CAD build for the part. Positions are in the model's coordinates, mm. A direction names the side the tool comes from. Coordinates: 2 decimals unless noted, no trailing zeros. Order: outer loops, then holes, each group sorted by start corner. A loop starts at its lowest first (then second) coordinate and runs counter-clockwise, first axis right, second up. Notation, with made-up numbers: (24, -25.75) - (38, -25.75) arc R21 ccw to (38, 6.25) - close; hole circle Ø9 at (55, 49). An arc over 180 degrees is marked (long way). Return JSON: item names as keys, results as strings.
from build123d import *

# Parameters (mm, degrees)
F0_W      = 93
F0_H      = 70
F0_R      = 1.5
F0_H_2    = 17
F0_R_2    = 3.25
F0_W_2    = 6
F0_H_3    = 6
F0_R_3    = 6
F0_W_3    = 14
F0_H_4    = 12
F0_R_4    = 3.5
F0_R_5    = 1.75
F1_DEPTH  = 1.5
F2_W      = 20.3
F2_H      = 8.7
F2_W_2    = 18.3
F2_H_2    = 6.7
F3_DEPTH  = 9
F2_W_3    = 26
F2_H_3    = 26.35
F4_DEPTH  = 3.5
F5_DEPTH  = 18.5
F6_DEPTH  = 6
F2_W_4    = 50
F2_H_4    = 1.5
F7_DEPTH  = 4
F8_DEPTH  = 10
F9_DEPTH  = 3.5
F10_DEPTH = 6.7
F11_DEPTH = 27
F12_DEPTH = 17
F13_DEPTH = 14
F14_DEPTH = 7
F15_DEPTH = 8
F16_W     = 6
F16_H     = 43
F17_DEPTH = 3.5
F18_DEPTH = 8
F19_R     = 1
F21_DEPTH = 1
F22_W     = 2.2
F22_H     = 24
F23_DEPTH = 10


with BuildPart() as f1:
    # F0 (on Front) → F1 (new body)
    with BuildSketch(Plane.XZ):
        with Locations((46.5, 52)):
            Rectangle(F0_W, F0_H)
        with Locations((2.5, 19.5)):
            Circle(F0_R, mode=Mode.SUBTRACT)
        with Locations((90.5, 19.5)):
            Circle(F0_R, mode=Mode.SUBTRACT)
        with Locations((2.5, 84.5)):
            Circle(F0_R, mode=Mode.SUBTRACT)
        with Locations((90.5, 84.5)):
            Circle(F0_R, mode=Mode.SUBTRACT)
        with Locations((46.5, 8.5)):
            Rectangle(F0_W, F0_H_2)
        with Locations((8.5, 11.5)):
            Circle(F0_R_2, mode=Mode.SUBTRACT)
        with Locations((50, 8)):
            Rectangle(F0_W_2, F0_H_3, mode=Mode.SUBTRACT)
        with Locations((65.5, 8)):
            Circle(F0_R_3, mode=Mode.SUBTRACT)
        with Locations((83, 8)):
            Rectangle(F0_W_3, F0_H_4, mode=Mode.SUBTRACT)
        with Locations((83, 8)):
            Rectangle(F0_W_3, F0_H_4)
        with Locations((83, 8)):
            Circle(F0_R_4, mode=Mode.SUBTRACT)
        with Locations((65.5, 8)):
            Circle(F0_R_3)
        with Locations((83, 8)):
            Circle(F0_R_4)
        with BuildLine():
            ThreePointArc((80.4019237886, 6.5), (82.2235428647, 10.8977774789), (86, 8))
            ThreePointArc((86, 8), (85.8977774789, 7.2235428647), (85.5980762114, 6.5))
            ThreePointArc((85.5980762114, 6.5), (83, 5), (80.4019237886, 6.5))
        make_face(mode=Mode.SUBTRACT)
        with Locations((50, 8)):
            Rectangle(F0_W_2, F0_H_3)
        with Locations((50, 8)):
            Circle(F0_R_5, mode=Mode.SUBTRACT)
        with Locations((8.5, 11.5)):
            Circle(F0_R_2)
        with BuildLine():
            ThreePointArc((85.5980762114, 6.5), (85.8977774789, 7.2235428647), (86, 8))
            ThreePointArc((86, 8), (82.2235428647, 10.8977774789), (80.4019237886, 6.5))
            Line((80.4019237886, 6.5), (85.5980762114, 6.5))
        make_face()
        with Locations((50, 8)):
            Circle(F0_R_5)
        with BuildLine():
            Line((85.5980762114, 6.5), (80.4019237886, 6.5))
            ThreePointArc((80.4019237886, 6.5), (83, 5), (85.5980762114, 6.5))
        make_face()
    extrude(amount=-F1_DEPTH)

    # F2 (on face) → F3 (join)
    with BuildSketch(Plane(origin=(0, 1.5, 0), x_dir=(-1, 0, 0), z_dir=(0, 1, 0))):
        with Locations((-61.75, 76.05)):
            Rectangle(F2_W, F2_H)
        with Locations((-61.75, 76.05)):
            Rectangle(F2_W_2, F2_H_2, mode=Mode.SUBTRACT)
        with Locations((-31.25, 76.05)):
            Rectangle(F2_W, F2_H)
        with Locations((-31.25, 76.05)):
            Rectangle(F2_W_2, F2_H_2, mode=Mode.SUBTRACT)
    extrude(amount=F3_DEPTH)

    # F2 (on face) → F4 (join)
    with BuildSketch(Plane(origin=(0, 1.5, 0), x_dir=(-1, 0, 0), z_dir=(0, 1, 0))):
        with Locations((-13, 51.525)):
            Rectangle(F2_W_3, F2_H_3)
    extrude(amount=F4_DEPTH)

    # F5 (add): faces of the model
    f5_faces = [f1.faces().sort_by_distance(p)[0] for p in [
        (61.75, 1.5, 76.05),
        (31.25, 1.5, 76.05),
    ]]
    extrude(f5_faces, amount=F5_DEPTH)

    # F0 (on Front) → F6 (join)
    with BuildSketch(Plane.XZ):
        with Locations((46.5, 52)):
            Rectangle(F0_W, F0_H)
        with Locations((2.5, 19.5)):
            Circle(F0_R, mode=Mode.SUBTRACT)
        with Locations((90.5, 19.5)):
            Circle(F0_R, mode=Mode.SUBTRACT)
        with Locations((2.5, 84.5)):
            Circle(F0_R, mode=Mode.SUBTRACT)
        with Locations((90.5, 84.5)):
            Circle(F0_R, mode=Mode.SUBTRACT)
    extrude(amount=F6_DEPTH)

    # F2 (on face) → F7 (join)
    with BuildSketch(Plane(origin=(0, 1.5, 0), x_dir=(-1, 0, 0), z_dir=(0, 1, 0))):
        with Locations((-38, 19.5)):
            Rectangle(F2_W_4, F2_H_4)
    extrude(amount=F7_DEPTH)

    # F0 (on Front) → F8 (join)
    with BuildSketch(Plane.XZ):
        with Locations((65.5, 8)):
            Circle(F0_R_3)
    extrude(amount=F8_DEPTH)

    # F0 (on Front) → F9 (join)
    with BuildSketch(Plane.XZ):
        with Locations((50, 8)):
            Rectangle(F0_W_2, F0_H_3)
        with Locations((50, 8)):
            Circle(F0_R_5, mode=Mode.SUBTRACT)
    extrude(amount=F9_DEPTH)

    # F0 (on Front) → F10 (join)
    with BuildSketch(Plane.XZ):
        with Locations((50, 8)):
            Circle(F0_R_5)
    extrude(amount=F10_DEPTH)

    # F0 (on Front) → F11 (join)
    with BuildSketch(Plane.XZ):
        with BuildLine():
            ThreePointArc((85.5980762114, 6.5), (85.8977774789, 7.2235428647), (86, 8))
            ThreePointArc((86, 8), (82.2235428647, 10.8977774789), (80.4019237886, 6.5))
            Line((80.4019237886, 6.5), (85.5980762114, 6.5))
        make_face()
    extrude(amount=F11_DEPTH)

    # F0 (on Front) → F12 (join)
    with BuildSketch(Plane.XZ):
        with BuildLine():
            Line((85.5980762114, 6.5), (80.4019237886, 6.5))
            ThreePointArc((80.4019237886, 6.5), (83, 5), (85.5980762114, 6.5))
        make_face()
    extrude(amount=F12_DEPTH)

    # F0 (on Front) → F13 (join)
    with BuildSketch(Plane.XZ):
        with Locations((83, 8)):
            Circle(F0_R_4)
        with BuildLine():
            ThreePointArc((80.4019237886, 6.5), (82.2235428647, 10.8977774789), (86, 8))
            ThreePointArc((86, 8), (85.8977774789, 7.2235428647), (85.5980762114, 6.5))
            ThreePointArc((85.5980762114, 6.5), (83, 5), (80.4019237886, 6.5))
        make_face(mode=Mode.SUBTRACT)
        with BuildLine():
            Line((85.5980762114, 6.5), (80.4019237886, 6.5))
            ThreePointArc((80.4019237886, 6.5), (83, 5), (85.5980762114, 6.5))
        make_face()
        with BuildLine():
            ThreePointArc((85.5980762114, 6.5), (85.8977774789, 7.2235428647), (86, 8))
            ThreePointArc((86, 8), (82.2235428647, 10.8977774789), (80.4019237886, 6.5))
            Line((80.4019237886, 6.5), (85.5980762114, 6.5))
        make_face()
    extrude(amount=F13_DEPTH)

    # F0 (on Front) → F14 (join)
    with BuildSketch(Plane.XZ):
        with Locations((83, 8)):
            Rectangle(F0_W_3, F0_H_4)
        with Locations((83, 8)):
            Circle(F0_R_4, mode=Mode.SUBTRACT)
    extrude(amount=F14_DEPTH)

    # F0 (on Front) → F15 (join)
    with BuildSketch(Plane.XZ):
        with Locations((8.5, 11.5)):
            Circle(F0_R_2)
    extrude(amount=F15_DEPTH)

    # F16 (on face) → F17 (join)
    with BuildSketch(Plane.XZ.offset(6)):
        with Locations((4.5, 52)):
            Rectangle(F16_W, F16_H)
    extrude(amount=F17_DEPTH)

    # F16 (on face) → F18 (join)
    with BuildSketch(Plane.XZ.offset(6)):
        Polygon((85.5, 77.5), (7.5, 77.5), (7.5, 73.5), (7.5, 30.5), (7.5, 26.5), (85.5, 26.5), align=None)
    extrude(amount=F18_DEPTH)

    # F19
    f19_edges = [f1.edges().sort_by_distance(p)[0] for p in [
        (7.5, -14, 52),
        (46.5, -14, 77.5),
        (46.5, -14, 26.5),
        (85.5, -14, 52),
        (7.5, -10, 26.5),
        (85.5, -10, 26.5),
        (7.5, -10, 77.5),
    ]]
    fillet(f19_edges, radius=F19_R)

    # F20 (on face) → F21 (cut)
    with BuildSketch(Plane.XZ.offset(14)):
        with BuildLine():
            Line((81.5, 72), (11.5, 72))
            ThreePointArc((11.5, 72), (10.7928932188, 71.7071067812), (10.5, 71))
            Line((10.5, 71), (10.5, 33))
            ThreePointArc((10.5, 33), (10.7928932188, 32.2928932188), (11.5, 32))
            Line((11.5, 32), (81.5, 32))
            ThreePointArc((81.5, 32), (82.2071067812, 32.2928932188), (82.5, 33))
            Line((82.5, 33), (82.5, 71))
            ThreePointArc((82.5, 71), (82.2071067812, 71.7071067812), (81.5, 72))
        make_face()
    extrude(amount=-F21_DEPTH, mode=Mode.SUBTRACT)

    # F22 (on face) → F23 (join)
    with BuildSketch(Plane(origin=(0, 0, 0), x_dir=(0, -1, 0), z_dir=(-1, 0, 0))):
        with Locations((-3.1, 51.525)):
            Rectangle(F22_W, F22_H)
    extrude(amount=F23_DEPTH)


solid = f1.part
Item 1: Band-saw the part on B-B, the plane x = 65.5. List the corners of the cut face in (y, z).
Findings below:
{"outline": "(-14, 27.5) arc R1 ccw to (-13, 26.5) - (-6, 26.5) - (-6, 17) - (0, 17) - (0, 14) - (-10, 14) - (-10, 2) - (0, 2) - (0, 0) - (1.5, 0) - (1.5, 71.7) - (10.5, 71.7) - (10.5, 72.7) - (20, 72.7) - (20, 79.4) - (10.5, 79.4) - (10.5, 80.4) - (1.5, 80.4) - (1.5, 87) - (-6, 87) - (-6, 77.5) - (-13, 77.5) arc R1 ccw to (-14, 76.5) - (-14, 72) - (-13, 72) - (-13, 32) - (-14, 32) - close"}
Item 2: Drop flat-ended pins along their axis: P1, Ø9.5, axis at y = 4, z = 75, coming from the -X side; P2, Ø5, axis at x = -5, z = 53, coming from the +Y side; P3, Ø1.5, axis at x = 75.5, z = 46.5, coming from the -Y side; P4, Ø1.8, axis at x = 2.5, z = 84.5, coming from the -Y side (3 decimals). Give the stop position or say it passes through.
Findings below:
{"P1": "stops at x = 0", "P2": "stops at y = 4.2", "P3": "stops at y = -13", "P4": "passes through"}
Item 3: Wall check: L1, parallel to Z at x = 90.5, y = -3; L2, parallel to Z at x = 90.5, y = 0.25; L3, parallel to X at y = -2, z = 84. Give the ranges that are in metal, low to high. Write a range as [from, to].
Findings below:
{"L1": "z = [17, 18], [21, 83], [86, 87]", "L2": "z = [0, 18], [21, 83], [86, 87]", "L3": "x = [0, 1.09], [3.91, 89.09], [91.91, 93]"}
Item 4: Mould opens along Z. For faces 1 (the flat face through (40.4, 15, 76)), 2 (the flat face through (46, -2, 87)), 3 (the cylindrical face through (86.233, -10.451, 6.659)) say: released by +Z, released by -Z, zero draft, split by the parting line, or undercut.
Findings below:
{"face 1": "zero draft", "face 2": "released by +Z", "face 3": "undercut"}
Item 5: Band-saw the part on A-A, the plane z = 84.5. List the corners of the cut face in (x, y).
Findings below:
{"outline": "(0, -6) - (1, -6) - (1, 1.5) - (0, 1.5) - close; (4, -6) - (89, -6) - (89, 1.5) - (4, 1.5) - close; (92, -6) - (93, -6) - (93, 1.5) - (92, 1.5) - close"}
Item 6: Band-saw the part on C-C, the plane z = 35. List the corners of the cut face in (x, y), then the cut area to 3 significant figures.
Findings below:
{"outline": "(0, -6) - (1.5, -6) - (1.5, -9.5) - (7.5, -9.5) - (7.5, -13) arc R1 ccw to (8.5, -14) - (10.5, -14) - (10.5, -13) - (82.5, -13) - (82.5, -14) - (84.5, -14) arc R1 ccw to (85.5, -13) - (85.5, -6) - (93, -6) - (93, 1.5) - (0, 1.5) - close", "area": "1,270 mm²"}
Item 7: Which spindle directions (+Z, -Z, +X, -X, +Y, -Y) get a long thin tool onto all of the face, cutting with end or side? Do faces 4 (the flat face through (1.5, -8, 52)), 5 (the flat face through (83, -7, 12)), 6 (the flat face through (13, 5, 52)). Say none if no direction does.
Findings below:
{"face 4": "+Z, -Z, -X, -Y", "face 5": "-Y", "face 6": "+X, -X, +Y"}
Item 8: Band-saw the part on D-D, the plane x = 50. List the corners of the cut face in (y, z).
Findings below:
{"outline": "(-14, 27.5) arc R1 ccw to (-13, 26.5) - (-6, 26.5) - (-6, 17) - (0, 17) - (0, 11) - (-3.5, 11) - (-3.5, 9.75) - (-6.7, 9.75) - (-6.7, 6.25) - (-3.5, 6.25) - (-3.5, 5) - (0, 5) - (0, 0) - (1.5, 0) - (1.5, 18.75) - (5.5, 18.75) - (5.5, 20.25) - (1.5, 20.25) - (1.5, 87) - (-6, 87) - (-6, 77.5) - (-13, 77.5) arc R1 ccw to (-14, 76.5) - (-14, 72) - (-13, 72) - (-13, 32) - (-14, 32) - close"}
